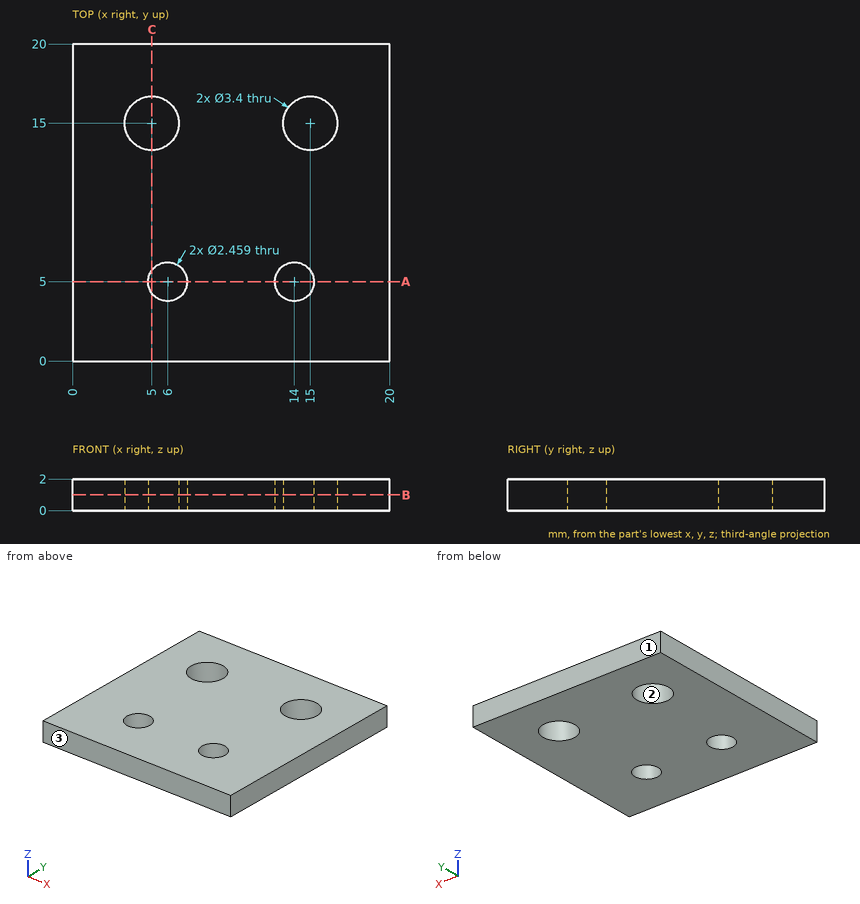
Verification items for this drawing (mm, ordinates from the low corner). Give positions to 0.01 mm unless a question says otherwise; leave off trailing zeros. Loops run counter-clockwise (first coordinate to the right, second up) from the corner with the lowest first, then second, coordinate; pieces in that order, holes last. Notation, with made-up numbers: M 83,-31 L 113,-31 A8 cw 113,-17 Z; hole C 73,29 d10. An arc over 180 degrees is marked long. Write item = value, one per line. Start each with the question number.
1. Thickness scan on probe 1 along X at (y, z) = (5, 1.1); probe 2 along Y at (x, z) = (14, 1.55); probe 3 along X at (y, z) = (15, 1.25). Record the ranges inside material, lowest first.
2. Section check C-C, the plane x = 5. Enter the section's corners in (y, z).
3. Section check B-B, the plane z = 1. Enter the section's corners in (x, y).
4. Go/stop test with a flat-tipped pin: P1, Ø2.5, axis at x = 5, y = 15, coming from the +Z side. Record where the tip stops, or that it passes through.
5. Draft check along Y on the marked faces 1, 2 and 3. Enter one of: +Y half, -Y half, draft (parallel to the pull), parting line (faces both ways), or undercut.
6. Section check A-A, the plane y = 5. Enter the section's corners in (x, z), plus the area to 3 significant figures.
Values follow:
q1.probe_1 = 0 to 4.77, 7.23 to 12.77, 15.23 to 20
q1.probe_2 = 0 to 3.77, 6.23 to 13.63, 16.37 to 20
q1.probe_3 = 0 to 3.3, 6.7 to 13.3, 16.7 to 20
q2.outline = M 0,0 L 4.28,0 L 4.28,2 L 0,2 Z; M 5.72,0 L 13.3,0 L 13.3,2 L 5.72,2 Z; M 16.7,0 L 20,0 L 20,2 L 16.7,2 Z
q3.outline = M 0,0 L 20,0 L 20,20 L 0,20 Z; hole C 5,15 d3.4; hole C 6,5 d2.46; hole C 14,5 d2.46; hole C 15,15 d3.4
q4.P1 = through
q5.face_1 = +Y half
q5.face_2 = undercut
q5.face_3 = -Y half
q6.outline = M 0,0 L 4.77,0 L 4.77,2 L 0,2 Z; M 7.23,0 L 12.77,0 L 12.77,2 L 7.23,2 Z; M 15.23,0 L 20,0 L 20,2 L 15.23,2 Z
q6.area = 30.2 mm^2
